Geometry check sheet. Reference: the model listing, model coordinates, mm. Face numbers are marked on the shaded views. Round coordinates to 2 decimals unless told otherwise and drop trailing zeros. Loops run counter-clockwise (first coordinate to the right, second up) from the corner with the lowest first, then second, coordinate; pieces in that order, holes last. Notation, with made-up numbers: (-40, 12.25) -> (-8, 12.25) arc R35 ccw to (-8, 49.25) -> close; hole circle Ø2 at (-29, 66). An arc over 180 degrees is marked (long way). Use a Markdown table: item, result. Add a question column.
Q1. Material ranges on L1, parallel to Y at x = 0, z = 1.05; L2, parallel to Y at x = -11.25, z = 0.4; L3, parallel to X at y = 6, z = 1.05, recorded low to high.
Q2. Gauge pin test, flat ends, axial feed: P1, Ø3.5, axis at x = -10.39, y = 0, coming from the -Z side; P2, Ø2.5, axis at x = 10.39, y = 0, coming from the +Z side. Record the tip position at first contact, or that the pin passes through.
Q3. Sectioned sample at A-A, the plane y = 0. Enter the section's corners in (x, z), then the cut area to 3 significant figures.
Q4. Sectioned sample at C-C, the plane x = 0. Enter the section's corners in (y, z).
Q5. Release check for a two-part mould opening along X. For the marked faces 1, 2 and 3 record: released by +X, released by -X, zero draft, split by the parting line, or undercut.
Q6. Sectioned sample at D-D, the plane y = 10. Enter the section's corners in (x, z).
Q7. Sectioned sample at B-B, the plane z = 0.6. Enter the section's corners in (x, y).
```python
from build123d import *

# Parameters (mm, degrees)
CYLINDER001_R     = 1
CYLINDER001_DEPTH = 10
CYLINDER_R        = 1
CYLINDER_DEPTH    = 10
SKETCH_R          = 1.5
PAD_DEPTH         = 1.66


with BuildPart() as cilindro001:
    # Cylinder001 → Cylinder001 (new body)
    with BuildSketch(Plane(origin=(0, 6, -2), x_dir=(1, 0, 0), z_dir=(0, 0, 1))):
        Circle(CYLINDER001_R)
    extrude(amount=CYLINDER001_DEPTH)


with BuildPart() as cilindro:
    # Cylinder → Cylinder (new body)
    with BuildSketch(Plane(origin=(0, 10, -2), x_dir=(1, 0, 0), z_dir=(0, 0, 1))):
        Circle(CYLINDER_R)
    extrude(amount=CYLINDER_DEPTH)


with BuildPart() as obj1:
    # Sketch → Pad (new body)
    with BuildSketch(Plane.XY):
        with BuildLine():
            Line((-13.856406, 2), (-8.660254, 11))
            ThreePointArc((-5.196152, 13), (-7.196152, 12.464102), (-8.660254, 11))
            Line((-5.196152, 13), (5.196152, 13))
            ThreePointArc((8.660254, 11), (7.196152, 12.464102), (5.196152, 13))
            Line((8.660254, 11), (13.856406, 2))
            ThreePointArc((13.856406, -2), (14.392305, 0), (13.856406, 2))
            Line((13.856406, -2), (8.660254, -11))
            ThreePointArc((5.196152, -13), (7.196152, -12.464102), (8.660254, -11))
            Line((5.196152, -13), (-5.196152, -13))
            ThreePointArc((-8.660254, -11), (-7.196152, -12.464102), (-5.196152, -13))
            Line((-8.660254, -11), (-13.856406, -2))
            ThreePointArc((-13.856406, 2), (-14.392305, 0), (-13.856406, -2))
        make_face()
        with Locations((-10.392305, 0)):
            Circle(SKETCH_R, mode=Mode.SUBTRACT)
        with Locations((10.392305, 0)):
            Circle(SKETCH_R, mode=Mode.SUBTRACT)
    extrude(amount=PAD_DEPTH)

    # Cut003: cut Cilindro
    add(cilindro.part, mode=Mode.SUBTRACT)

    # Cut004: cut Cilindro001
    add(cilindro001.part, mode=Mode.SUBTRACT)


solid = obj1.part
```
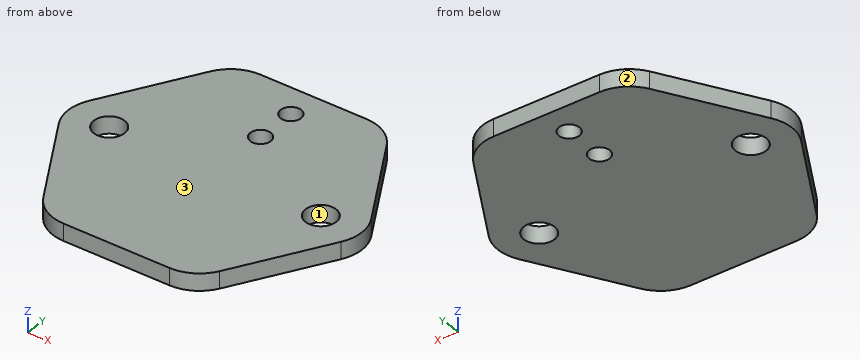
Values:
| question | item | result |
|---|---|---|
| 1 | L1 | -13 to 5, 7 to 9, 11 to 13 |
| 1 | L2 | -6.51 to -1.23, 1.23 to 6.51 |
| 1 | L3 | -11.55 to -1, 1 to 11.55 |
| 2 | P1 | z = 0 |
| 2 | P2 | through |
| 3 | outline | (-14.39, 0) -> (-11.89, 0) -> (-11.89, 1.66) -> (-14.39, 1.66) -> close; (-8.89, 0) -> (8.89, 0) -> (8.89, 1.66) -> (-8.89, 1.66) -> close; (11.89, 0) -> (14.39, 0) -> (14.39, 1.66) -> (11.89, 1.66) -> close |
| 3 | area | 37.8 mm^2 |
| 4 | outline | (-13, 0) -> (5, 0) -> (5, 1.66) -> (-13, 1.66) -> close; (7, 0) -> (9, 0) -> (9, 1.66) -> (7, 1.66) -> close; (11, 0) -> (13, 0) -> (13, 1.66) -> (11, 1.66) -> close |
| 5 | face 1 | undercut |
| 5 | face 2 | released by -X |
| 5 | face 3 | zero draft |
| 6 | outline | (-9.24, 0) -> (-1, 0) -> (-1, 1.66) -> (-9.24, 1.66) -> close; (1, 0) -> (9.24, 0) -> (9.24, 1.66) -> (1, 1.66) -> close |
| 7 | outline | (-13.86, -2) -> (-8.66, -11) arc R4 ccw to (-5.2, -13) -> (5.2, -13) arc R4 ccw to (8.66, -11) -> (13.86, -2) arc R4 ccw to (13.86, 2) -> (8.66, 11) arc R4 ccw to (5.2, 13) -> (-5.2, 13) arc R4 ccw to (-8.66, 11) -> (-13.86, 2) arc R4 ccw to start; hole circle Ø3 at (-10.39, 0); hole circle Ø2 at (0, 6); hole circle Ø2 at (0, 10); hole circle Ø3 at (10.39, 0) |
